from build123d import *

# Parameters (mm, degrees)
SCHIZZO2_W                   = 30
SCHIZZO2_H                   = 30
SCHIZZO2_R                   = 7.5
ESTRUSIONE_ESTRUSIONE1_DEPTH = 30
SCHIZZO3_R                   = 4
TAGLIO_ESTRUSIONE1_DEPTH     = 13
SCHIZZO5_R                   = 4
TAGLIO_ESTRUSIONE2_DEPTH     = 12


with BuildPart() as part:
    # Schizzo2 → Estrusione-Estrusione1 (new body)
    with BuildSketch(Plane.XY):
        Rectangle(SCHIZZO2_W, SCHIZZO2_H)
        with Locations((1.8, 3)):
            Circle(SCHIZZO2_R, mode=Mode.SUBTRACT)
    extrude(amount=-ESTRUSIONE_ESTRUSIONE1_DEPTH)

    # Schizzo3 → Taglio-Estrusione1 (cut)
    with BuildSketch(Plane.ZY.offset(15)):
        with Locations((-15, -5)):
            Circle(SCHIZZO3_R)
    extrude(amount=-TAGLIO_ESTRUSIONE1_DEPTH, mode=Mode.SUBTRACT)

    # Schizzo5 → Taglio-Estrusione2 (cut)
    with BuildSketch(Plane.XZ.offset(15)):
        with Locations(Location((5, -15, 0), (0, 0, 270))):
            Circle(SCHIZZO5_R)
    extrude(amount=-TAGLIO_ESTRUSIONE2_DEPTH, mode=Mode.SUBTRACT)


solid = part.part
Geometry check sheet. Reference: the model listing, model coordinates, mm. A direction names the side the tool comes from. Coordinates: 2 decimals unless noted, no trailing zeros. Loops run counter-clockwise (first coordinate to the right, second up) from the corner with the lowest first, then second, coordinate; pieces in that order, holes last. Notation, with made-up numbers: (-6, 3.25) - (0, 3.25) arc R27 cw to (0, 36.25) - close; hole circle Ø9 at (-26, 84.5). An arc over 180 degrees is marked (long way). Use one line per item in the form item = value. Start each with the question number.
Item 1: Mould release check, pull along Z, two halves, no side actions. Record for faces 1 (the face through (-4, -3, -30)), 2 (the face through (0, -15, -15)), 3 (the face through (8.966, -9.084, -14.479)): +Z half, -Z half, draft (parallel to the pull), parting line (faces both ways), or undercut.
Item 2: Section check D-D, the plane y = 8. Enter the section's corners in (x, z), and give its area (3 significant figures).
Item 3: Thickness scan on probe 1 along Z at (x, y) = (5, -6); probe 2 along Y at (x, z) = (-4.75, -15); probe 3 along Y at (x, z) = (-12, -15). Record the ranges inside material, lowest first.
Item 4: Section check C-C, the plane z = -15. Enter the section's corners in (x, y), and give its area (3 significant figures).
Item 5: Tool access check on faces 4 (the face through (-4, -3, 0)), 5 (the face through (-8.591, -8.905, -15.867)). Record the directions out of +Z, -Z, +X, -X, +Y, -Y that give a thin tool (end or side, any length) a straight path to the whole face; none if there is none.
Item 6: Section check A-A, the plane x = 1.8. Enter the section's corners in (y, z).
Item 7: Gauge pin test, flat ends, axial feed: pin 1 (5 mm diameter, centred on y = -5, z = -15, fed in from -X); pin 2 (1.4 mm diameter, centred on x = 7.5, z = -16, fed in from -Y). Record the tip position at first contact, or that the pin passes through.
Item 8: Section check B-B, the plane y = -5. Enter the section's corners in (x, z).
Computed:
q1.face_1 = -Z half
q1.face_2 = draft
q1.face_3 = undercut
q2.outline = (-15, -30) - (-3.79, -30) - (-3.79, 0) - (-15, 0) - close; (7.39, -30) - (15, -30) - (15, 0) - (7.39, 0) - close
q2.area = 565 mm2
q3.probe_1 = -30 to -19, -11 to 0
q3.probe_2 = -15 to -9, -1 to -0.65, 6.65 to 15
q3.probe_3 = -15 to -9, -1 to 15
q4.outline = (-15, -15) - (1, -15) - (1, -4.46) arc R7.5 cw to (-2, -3.47) - (-2, -9) - (-15, -9) - close; (-15, -1) - (-4.54, -1) arc R7.5 cw (long way) to (6.3, -3) - (9, -3) - (9, -15) - (15, -15) - (15, 15) - (-15, 15) - close
q4.area = 533 mm2
q5.face_4 = +Z, +X, -X, +Y, -Y
q5.face_5 = -X
q6.outline = (-15, -30) - (-4.5, -30) - (-4.5, -17.4) - (-15, -17.4) - close; (-15, -12.6) - (-4.5, -12.6) - (-4.5, 0) - (-15, 0) - close; (10.5, -30) - (15, -30) - (15, 0) - (10.5, 0) - close
q7.pin_1 = -2
q7.pin_2 = -3
q8.outline = (-15, -30) - (15, -30) - (15, 0) - (-15, 0) - (-15, -11) - (-2, -11) - (-2, -19) - (-15, -19) - close; hole circle Ø8 at (5, -15)
